Autodesk Inventor part; units mm, degrees
ref_plane "YZ Plane" through (0, 0, 0) normal (1, 0, 0) x (0, 1, 0)
ref_plane "XZ Plane" through (0, 0, 0) normal (0, 1, 0) x (-1, 0, 0)
ref_plane "XY Plane" through (0, 0, 0) normal (0, 0, 1) x (1, 0, 0)
sketch "Sketch1" plane through (0, 0, 0) normal (0, 1, 0) x (-1, 0, 0)
  line L0 (0, 0) -> (-50, 0)
  line L1 (-50, 0) -> (-50, 80)
  line L2 (-50, 80) -> (0, 80)
  line L3 (0, 80) -> (0, 0)
  dimension "d0" = 50
  dimension "d1" = 80
extrude "Extrusion1" add sketch "Sketch1" along normal blind 1.6
sketch "Sketch2" plane through (0, 1.6, 0) normal (0, 1, 0) x (1, 0, 0)
  circle A0 centre (10.152, -55.746) radius 4
  line L0 (0, 0) -> (0, -80)
  line L1 (50, 0) -> (0, 0)
  line L2 (0, -80) -> (50, -80)
  circle A1 centre (39.85, -55.746) radius 4
  circle A2 centre (25, -19.9) radius 4
  point P0 (25, -80)
  dimension "d4" = 10.152
  dimension "d5" = 8
  dimension "d9" = 24.254
  dimension "d10" = 8
  dimension "d11" = 29.698
  dimension "d12" = 8
  dimension "d13" = 19.9
extrude "Holes for" cut sketch "Sketch2" against normal blind 10
equation "\"d12\" = d10"
properties part number "2020-04-02-10-10401-Outline_ConnectorPCB" material "ABS Plastic"
Verification items for the finished model (mm, model axes). Coordinates: 2 decimals unless noted, no trailing zeros. Loops run counter-clockwise (first coordinate to the right, second up) from the corner with the lowest first, then second, coordinate; pieces in that order, holes last. Notation, with made-up numbers: (26.25, 76.5) - (43.25, 76.5) arc R20 ccw to (43.25, 80.5) - close; hole circle Ø10 at (0.5, 84). An arc over 180 degrees is marked (long way). Return JSON: item names as keys, results as strings.
1. Section check C-C, the plane y = 0.85. Record the boundary of the cut face in (x, z), then the cut area to 3 significant figures.
Established:
{"outline": "(0, 0) - (50, 0) - (50, 80) - (0, 80) - close; hole circle Ø8 at (10.15, 55.75); hole circle Ø8 at (25, 19.9); hole circle Ø8 at (39.85, 55.75)", "area": "3,850 mm2"}
2. Section check B-B, the plane x = 39.85. Record the boundary of the cut face in (y, z), then the cut area to 3 significant figures.
Established:
{"outline": "(0, 0) - (1.6, 0) - (1.6, 51.75) - (0, 51.75) - close; (0, 59.75) - (1.6, 59.75) - (1.6, 80) - (0, 80) - close", "area": "115 mm2"}
3. Thickness scan on L1, parallel to Z at x = 39.85, y = 0.8; L2, parallel to X at y = 1.55, z = 58.5; L3, parallel to Z at x = 25, y = 1.1. Record the ranges inside material, lowest first.
Established:
{"L1": "z = 0 to 51.75, 59.75 to 80", "L2": "x = 0 to 7.25, 13.05 to 36.95, 42.75 to 50", "L3": "z = 0 to 15.9, 23.9 to 80"}
4. Go/stop test with a flat-tipped pin: pin 1 (6.5 mm diameter, centred on x = 39.85, z = 55.746, fed in from +Y). Record where the tip stops, or that it passes through.
Established:
{"pin 1": "passes through"}
5. Mould release check, pull along X, two halves, no side actions. Record for faces 1 (the flat face through (25, 1, 0)), 2 (the cylindrical face through (9.63, 0.81, 51.78)), 3 (the flat face through (50, 1, 39)): +X half, -X half, draft (parallel to the pull), parting line (faces both ways), or undercut.
Established:
{"face 1": "draft", "face 2": "undercut", "face 3": "+X half"}
6. Section check A-A, the plane z = 19.9. Record the boundary of the cut face in (x, y), then the cut area to 3 significant figures.
Established:
{"outline": "(0, 0) - (21, 0) - (21, 1.6) - (0, 1.6) - close; (29, 0) - (50, 0) - (50, 1.6) - (29, 1.6) - close", "area": "67.2 mm2"}
